```python
from build123d import *

# Parameters (mm, degrees)
BOSS_EXTRU_2_DEPTH      = 10
ESQUISSE3_R             = 1.25
ENL_V_MAT_EXTRU_1_DEPTH = 10
CONG_1_R                = 2
CONG_2_R                = 2
CONG_3_R                = 2
CONG_4_R                = 2


with BuildPart() as part:
    # Esquisse2 → Boss.-Extru.2 (new body)
    with BuildSketch(Plane.XY):
        Polygon((0, 0), (85, 0), (146.059462923, -38.154187025), (133.338741481, -38.154187025), (133.338741481, -35.205398061), (85, -5), (0, -5), (-48.338741481, -35.205398061), (-48.338741481, -38.154187025), (-61.059462923, -38.154187025), align=None)
    extrude(amount=BOSS_EXTRU_2_DEPTH)

    # Esquisse3 → Enlèv. mat.-Extru.1 (cut)
    with BuildSketch(Plane(origin=(0, 0, 0), x_dir=(1, 0, 0), z_dir=(0, 1, 0))):
        with Locations(Location((77, -5, 0), (0, 0, 270))):
            Circle(ESQUISSE3_R)
        with Locations(Location((8, -5, 0), (0, 0, 270))):
            Circle(ESQUISSE3_R)
    extrude(amount=-ENL_V_MAT_EXTRU_1_DEPTH, mode=Mode.SUBTRACT)

    # Congé1
    cong_1_edges = [part.edges().sort_by_distance(p)[0] for p in [
        (42.5, -5, 10),
    ]]
    fillet(cong_1_edges, radius=CONG_1_R)

    # Congé2
    cong_2_edges = [part.edges().sort_by_distance(p)[0] for p in [
        (107.569036211, -19.102699031, 10),
        (109.16937074, -20.102699031, 0),
        (-22.569036211, -19.102699031, 10),
        (-24.16937074, -20.102699031, 0),
        (42.5, -5, 0),
    ]]
    fillet(cong_2_edges, radius=CONG_2_R)

    # Congé3
    cong_3_edges = [part.edges().sort_by_distance(p)[0] for p in [
        (-61.059462923, -38.154187025, 5),
    ]]
    fillet(cong_3_edges, radius=CONG_3_R)

    # Congé4
    cong_4_edges = [part.edges().sort_by_distance(p)[0] for p in [
        (146.059462923, -38.154187025, 5),
    ]]
    fillet(cong_4_edges, radius=CONG_4_R)


solid = part.part
```
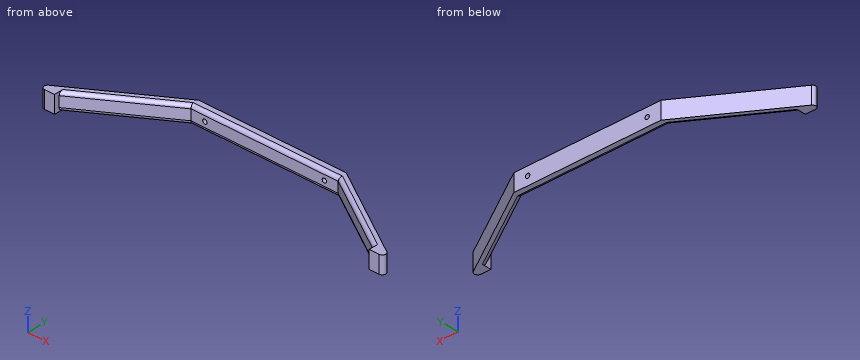
CAD build for the part. Positions are in the model's coordinates, mm. Coordinates: 2 decimals unless noted, no trailing zeros. Order: outer loops, then holes, each group sorted by start corner. A loop starts at its lowest first (then second) coordinate and runs counter-clockwise, first axis right, second up.
(1) Drill centre lines: L1, parallel to Z at x = 77, y = -2.85; L2, parallel to X at y = -3.2, z = 5; L3, parallel to X at y = -3.75, z = 5. Where is each one in solid material? Low to high.
Solution:
L1: z = 0 to 3.75, 6.25 to 10
L2: x = -5.12 to 6.75, 9.25 to 75.75, 78.25 to 90.12
L3: x = -6 to 6.75, 9.25 to 75.75, 78.25 to 91
(2) Saw through at A-A, the plane x = 18.5. Write the cut outline in (y, z), and give its area (3 significant figures).
Solution:
outline: (-5, 2) arc R2 ccw to (-3, 0) - (0, 0) - (0, 10) - (-3, 10) arc R2 ccw to (-5, 8) - close
area: 48.3 mm2
(3) Pin check, flat tips, straight feed: pin 1 Ø1.5 at (x, z) = (2, 7.5) entering from -Y; pin 2 Ø2 at (y, z) = (-32.5, 6.5) entering from -X; pin 3 Ø6 at (x, y) = (107, -23.5) entering from +Z; pin 4 Ø1.6 at (y, z) = (-36.5, 3.5) entering from +X. Stop position of each tip, or through.
Solution:
pin 1: stops at y = -5
pin 2: stops at x = -53.61
pin 3: passes through
pin 4: stops at x = 141.08
